Source: three-view drawing plus pictorial views. Frame: mm from the lowest corner of the part. Coordinates: 2 decimals unless noted, no trailing zeros. Order: outer loops, then holes, each group sorted by start corner. A loop starts at its lowest first (then second) coordinate and runs counter-clockwise, first axis right, second up. Notation, with made-up numbers: (55, -15) -> (90, -15) arc R29 ccw to (90, 21) -> close; hole circle Ø7 at (81, -23.75). An arc over 180 degrees is marked (long way). Use CSV: the item, a comma, the result in double quotes. Start each with the question number.
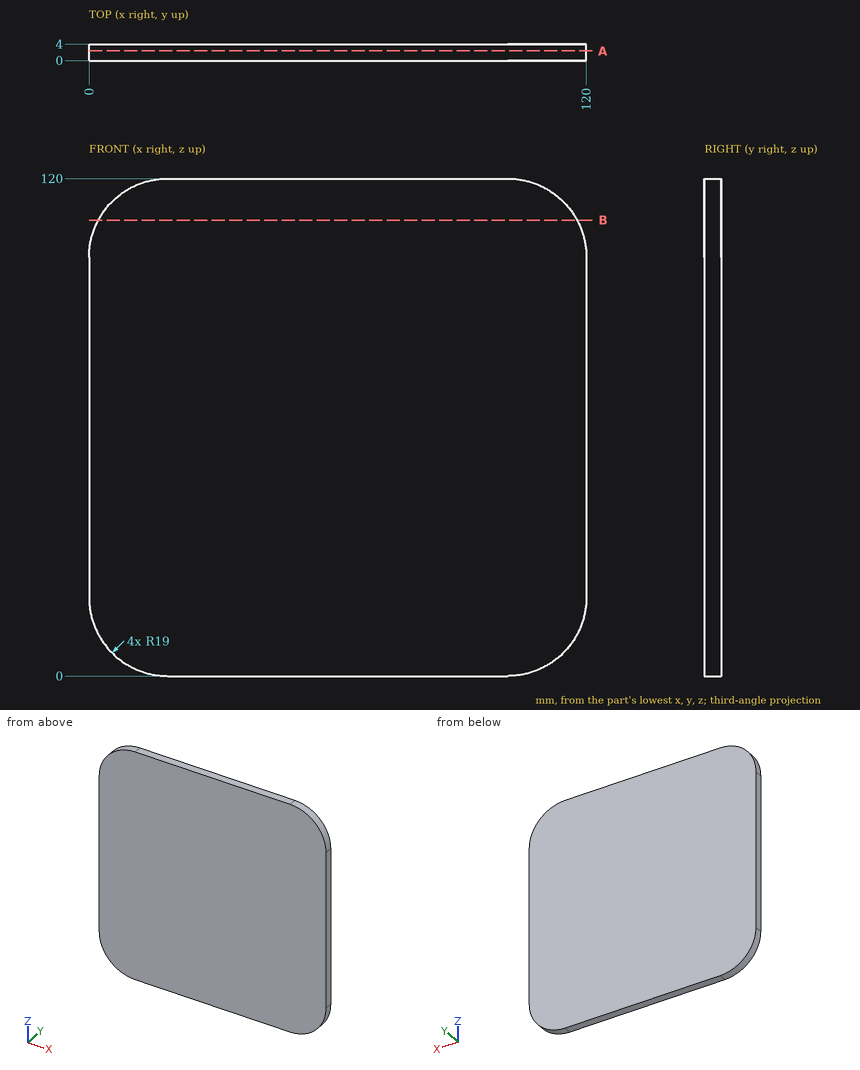
1. Section B-B on z = 110. Return loops of the section in (x, y), then the cut area to 3 significant figures.
2. Material intervals for line 1 along X through (y, z) = (1.3, 110); line 2 along X through (y, z) = (2.1, 106), sorted ascending.
3. Section A-A on y = 2.35. Return loops of the section in (x, z), then the cut area to 3 significant figures.
4. Contact query for a flat-ended pin moving along its axis: P1, Ø1.5, axis at x = 42, y = 2.5, coming from the -Z side. Output: stop coordinate, or through.
Values follow:
1,outline,"(2.27, 0) -> (117.73, 0) -> (117.73, 4) -> (2.27, 4) -> close"
1,area,"462 mm2"
2,line 1,"x = 2.27 to 117.73"
2,line 2,"x = 0.67 to 119.33"
3,outline,"(0, 19) arc R19 ccw to (19, 0) -> (101, 0) arc R19 ccw to (120, 19) -> (120, 101) arc R19 ccw to (101, 120) -> (19, 120) arc R19 ccw to (0, 101) -> close"
3,area,"14,100 mm2"
4,P1,"stops at z = 0"
